For this review, use the dimensioned drawing (mm, ordinates from the lowest corner) and the shaded views. Coordinates: 2 decimals unless noted, no trailing zeros. Write each loop counter-clockwise with the first axis right and the second up, starting at its lowest first coordinate (ties: lowest second). Pieces come first, ordered by that corner, then holes. Notation, with made-up numbers: (63.25, 13.5) - (119.25, 13.5) arc R30 cw to (119.25, 45.5) - close; hole circle Ø2 at (52, 67.5). An arc over 180 degrees is marked (long way). Use one line per item in the form item = value. Start each with the question number.
1) We need section D-D (z = 53). Give the boundary of the cut face in (x, y).
2) Insertion check: P1, Ø1.9, axis at x = 2, z = 74.5, coming from the -Y side; P2, Ø1.9, axis at x = 4.5, y = 7, coming from the +Z side; P3, Ø3, axis at x = 3, z = 46.5, coming from the -Y side. Each pin has a flat end and moves straight along its axis. Give the tip position at first contact, or say it passes through.
3) We need section C-C (x = 2.25). Give the boundary of the cut face in (y, z) (3 decimals), plus the area to 3 significant figures.
4) For L1, parallel to Z at x = 3.5, y = 48 (3 decimals); L2, parallel to Y at x = 4.75, z = 33.5; L3, parallel to Y at x = 1.75, z = 72, list the stretches that pass through material, from the lowest coordinate up. Write a range as from..to.
5) We need section A-A (z = 7.5). Give the boundary of the cut face in (x, y).
6) We need section B-B (y = 20). Give the boundary of the cut face in (x, z) (3 decimals), plus the area to 3 significant figures.
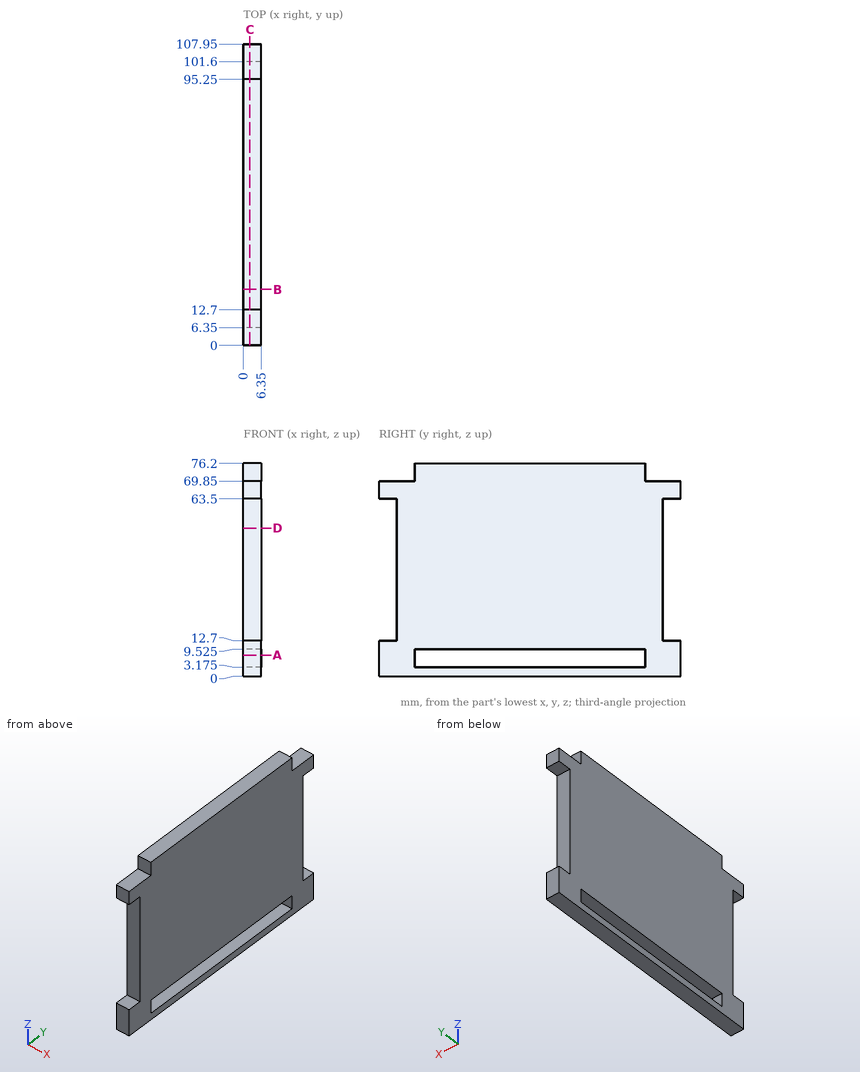
Determined:
q1.outline = (0, 6.35) - (6.35, 6.35) - (6.35, 101.6) - (0, 101.6) - close
q2.P1 = 12.7
q2.P2 = 69.85
q2.P3 = 6.35
q3.outline = (0, 0) - (107.95, 0) - (107.95, 12.7) - (101.6, 12.7) - (101.6, 63.5) - (107.95, 63.5) - (107.95, 69.85) - (95.25, 69.85) - (95.25, 76.2) - (12.7, 76.2) - (12.7, 69.85) - (0, 69.85) - (0, 63.5) - (6.35, 63.5) - (6.35, 12.7) - (0, 12.7) - close; hole (12.7, 3.175) - (95.25, 3.175) - (95.25, 9.525) - (12.7, 9.525) - close
q3.area = 6,900 mm²
q4.L1 = 0..3.175, 9.525..76.2
q4.L2 = 6.35..101.6
q4.L3 = 12.7..95.25
q5.outline = (0, 0) - (6.35, 0) - (6.35, 12.7) - (0, 12.7) - close; (0, 95.25) - (6.35, 95.25) - (6.35, 107.95) - (0, 107.95) - close
q6.outline = (0, 0) - (6.35, 0) - (6.35, 3.175) - (0, 3.175) - close; (0, 9.525) - (6.35, 9.525) - (6.35, 76.2) - (0, 76.2) - close
q6.area = 444 mm²
